from build123d import *

# Parameters (mm, degrees)
FILLET2_R          = 2
FILLET3_R          = 2
SKETCH2_R          = 2.95
CUT_EXTRUDE1_DEPTH = 13


with BuildPart() as part:
    # Sketch1 → Revolve1 (revolve)
    with BuildSketch(Plane.XY, mode=Mode.PRIVATE) as revolve1_sk:
        Polygon((-12.309472934, 14.722222222), (-27.309472934, 14.722222222), (-27.309472934, -19.777777778), (-32.309472934, -19.777777778), (-32.309472934, 19.722222222), (-12.309472934, 19.722222222), align=None)
    revolve(revolve1_sk.sketch.rotate(Axis((-53.278814679, -29.777777778, 0), (1, 0, 0)), 90), axis=Axis((-53.278814679, -29.777777778, 0), (1, 0, 0)))

    # Fillet2
    fillet2_edges = [part.edges().sort_by_distance(p)[0] for p in [
        (-32.309472934, -29.777777778, -49.5),
    ]]
    fillet(fillet2_edges, radius=FILLET2_R)

    # Fillet3
    fillet3_edges = [part.edges().sort_by_distance(p)[0] for p in [
        (-12.309472934, -29.777777778, -49.5),
    ]]
    fillet(fillet3_edges, radius=FILLET3_R)

    # Sketch2 → Cut-Extrude1 (cut, symmetric)
    with BuildSketch(Plane(origin=(-27.309472934, 0, 0), x_dir=(0, 0, -1), z_dir=(1, 0, 0))):
        with Locations((0, -11.277777778)):
            Circle(SKETCH2_R)
    extrude(amount=CUT_EXTRUDE1_DEPTH, both=True, mode=Mode.SUBTRACT)


solid = part.part
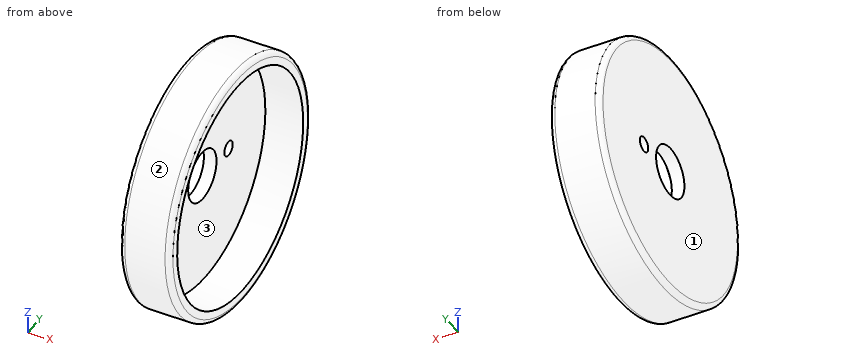
CAD build for the part. Positions are in the model's coordinates, mm. Face numbers are marked on the shaded views. Round coordinates to 2 decimals unless told otherwise and drop trailing zeros. Write each loop counter-clockwise with the first axis right and the second up, starting at its lowest first coordinate (ties: lowest second). Pieces come first, ordered by that corner, then holes. Notation, with made-up numbers: (-17, 16) -> (9, 16) arc R23 cw to (9, 46) -> close; hole circle Ø11 at (11.25, -1.75). An arc over 180 degrees is marked (long way). Answer as a JSON object with one key per item and string values.
(1) Band-saw the part on B-B, the plane x = -29. List the corners of the cut face in (y, z).
Reported:
{"outline": "circle Ø99 at (-29.78, 0); hole circle Ø20 at (-29.78, 0); hole circle Ø5.9 at (-11.28, 0)"}
(2) Pin check, flat tips, straight feed: P1, Ø1, axis at y = -10, z = 14.5, coming from the +X side; P2, Ø5, axis at x = -21, y = -2.5, coming from the +Z side; P3, Ø10, axis at x = -22, y = 6.5, coming from the +Z side; P4, Ø4.5, axis at y = -11.28, z = 0, coming from the +X side. Stop position of each tip, or through.
Reported:
{"P1": "stops at x = -27.31", "P2": "stops at z = 42.85", "P3": "stops at z = 38.37", "P4": "passes through"}
(3) Two-plate mould, pull along Z, no slides. Class the marked faces 1, 2 and 3: +Z half, -Z half, draft (parallel to the pull), parting line (faces both ways), or undercut.
Reported:
{"face 1": "draft", "face 2": "parting line", "face 3": "undercut"}
(4) Probe probe 1 along Y at (x, z) = (-28.75, 0); probe 2 along X at (y, z) = (7.5, -11); probe 3 along Z at (x, y) = (-20, -68). List the from-to ranges inside material, lowest first. Write a range as [from, to].
Reported:
{"probe 1": "y = [-79.28, -39.78], [-19.78, -14.23], [-8.33, 19.72]", "probe 2": "x = [-32.31, -27.31]", "probe 3": "z = [-31.45, -22.79], [22.79, 31.45]"}
(5) Band-saw the part on A-A, the plane z = 0. List the corners of the cut face in (x, y), then the cut area to 3 significant figures.
Reported:
{"outline": "(-32.31, -77.28) arc R2 ccw to (-30.31, -79.28) -> (-14.31, -79.28) arc R2 ccw to (-12.31, -77.28) -> (-12.31, -74.28) -> (-27.31, -74.28) -> (-27.31, -39.78) -> (-32.31, -39.78) -> close; (-32.31, -19.78) -> (-27.31, -19.78) -> (-27.31, -14.23) -> (-32.31, -14.23) -> close; (-32.31, -8.33) -> (-27.31, -8.33) -> (-27.31, 14.72) -> (-12.31, 14.72) -> (-12.31, 17.72) arc R2 ccw to (-14.31, 19.72) -> (-30.31, 19.72) arc R2 ccw to (-32.31, 17.72) -> close", "area": "512 mm^2"}
(6) Band-saw the part on C-C, the plane x = -19. List the corners of the cut face in (y, z), then the cut area to 3 significant figures.
Reported:
{"outline": "circle Ø99 at (-29.78, 0); hole circle Ø89 at (-29.78, 0)", "area": "1,480 mm^2"}
